Read the model definition and answer for the solid it produces. Units are mm, in the model's axes. A direction names the side the tool comes from. Give positions to 0.01 mm unless a question says otherwise; leave off trailing zeros. Order: outer loops, then holes, each group sorted by start corner. A loop starts at its lowest first (then second) coordinate and runs counter-clockwise, first axis right, second up.
```python
from build123d import *

# Parameters (mm, degrees)
F0_W     = 30
F0_H     = 40
F1_DEPTH = 5
F2_R     = 1
F3_W     = 26
F3_H     = 36
F3_W_2   = 23
F3_H_2   = 1.5
F4_DEPTH = 12


with BuildPart() as f1:
    # F0 (on Top) → F1 (new body)
    with BuildSketch(Plane.XY):
        Rectangle(F0_W, F0_H)
    extrude(amount=F1_DEPTH)

    # F2
    f2_edges = [f1.edges().sort_by_distance(p)[0] for p in [
        (0, -20, 0),
        (15, 0, 0),
        (0, 20, 0),
        (-15, 0, 0),
    ]]
    fillet(f2_edges, radius=F2_R)

    # F3 (on face) → F4 (join)
    with BuildSketch(Plane.XY.offset(5)):
        Rectangle(F3_W, F3_H)
        Polygon((-11.5, 16.5), (11.5, 16.5), (11.5, 0.75), (11.5, -0.75), (11.5, -16.5), (-11.5, -16.5), (-11.5, -0.75), (-11.5, 0.75), align=None, mode=Mode.SUBTRACT)
        Rectangle(F3_W_2, F3_H_2)
    extrude(amount=F4_DEPTH)

    # F6: sweep along a path in F6_path
    with BuildLine(Plane(origin=(-13, 18, 17), x_dir=(0, -1, 0), z_dir=(0, 0, -1))) as f6_path:
        Line((0, 0), (36, 0))
        Line((36, 0), (36, -26))
        Line((36, -26), (0, -26))
        Line((0, -26), (0, 0))
    # F5 (on face) → F6 (sweep)
    with BuildSketch(Plane.XZ.offset(18)):
        Polygon((-14.5, 8), (-13, 7), (-13, 9), align=None)
        Polygon((-14.5, 11), (-13, 10), (-13, 12), align=None)
        Polygon((-14.5, 14), (-13, 13), (-13, 15), align=None)
    sweep(path=f6_path.line, transition=Transition.RIGHT)


solid = f1.part
```
1) For a pull along Z with two mould halves and no side action, classify faces 6 (the face through (-0.203, 18.76, 7.507)), 7 (the face through (0, -18, 6)), 8 (the face through (0, -16.5, 11)), 9 (the face through (-1, 0, 17)) as released by +Z, released by -Z, zero draft, split by the parting line, or undercut.
Final values:
face 6: undercut
face 7: undercut
face 8: zero draft
face 9: released by +Z
2) Given pin 1 (0.8 mm diameter, centred on y = -8.5, z = 12.5, fed in from -X); pin 2 (6 mm diameter, centred on y = 12.5, z = 13.5, fed in from -X); pin 3 (1.1 mm diameter, centred on y = -7.5, z = 9.5, fed in from +X) (3 decimals); pin 4 (12.5 mm diameter, centred on x = -5.5, y = 8.5, fed in from +Z), each flat-ended and moving along its own axis, determine where each tip first touches the part or whether it passes through.
Final values:
pin 1: stops at x = -13
pin 2: stops at x = -14.5
pin 3: stops at x = 13.075
pin 4: stops at z = 17
3) The part is cut by section B-B on x = -12.5. Determine the outline of the cut face in (y, z).
Final values:
outline: (-20, 1) arc R1 ccw to (-19, 0) - (19, 0) arc R1 ccw to (20, 1) - (20, 5) - (18, 5) - (18, 7) - (19.5, 8) - (18, 9) - (18, 10) - (19.5, 11) - (18, 12) - (18, 13) - (19.5, 14) - (18, 15) - (18, 17) - (-18, 17) - (-18, 15) - (-19.5, 14) - (-18, 13) - (-18, 12) - (-19.5, 11) - (-18, 10) - (-18, 9) - (-19.5, 8) - (-18, 7) - (-18, 5) - (-20, 5) - close
4) The part is cut by section A-A on z = 9.5. Determine the outline of the cut face in (x, y).
Final values:
outline: (-13, -18) - (13, -18) - (13, 18) - (-13, 18) - close; hole (-11.5, -16.5) - (11.5, -16.5) - (11.5, -0.75) - (-11.5, -0.75) - close; hole (-11.5, 0.75) - (11.5, 0.75) - (11.5, 16.5) - (-11.5, 16.5) - close
5) A tool of negligible diameter and unlimited length cuts with its end or side. For faces 1 (the face through (0, -20, 3)), 2 (the face through (13.76, 0.273, 10.507)), 3 (the face through (-0.203, 18.76, 13.507)), 4 (the face through (0, 9, 5)), 5 (the face through (0.203, -18.76, 10.507)), from which of +Z, -Z, +X, -X, +Y, -Y can it reach the whole face along a straight path? Write none if from no direction.
Final values:
face 1: +Z, -Z, +X, -X, -Y
face 2: +X, +Y, -Y
face 3: +X, -X, +Y
face 4: +Z
face 5: +X, -X, -Y
6) Consider L1, parallel to Y at x = -6.25, z = 5.25; L2, parallel to Y at x = 2.25, z = 11.75 (3 decimals); L3, parallel to Z at x = 13.25, y = -17. Determine where each line is inside the solid, lowest interval first.
Final values:
L1: y = -18 to -16.5, -0.75 to 0.75, 16.5 to 18
L2: y = -18.375 to -16.5, -0.75 to 0.75, 16.5 to 18.375
L3: z = 0 to 5, 7.17 to 8.83, 10.17 to 11.83, 13.17 to 14.83
